Check sheet for the modelled part. Datum: model origin and axes. Units: mm. A direction names the side the tool comes from. Give positions to 0.01 mm unless a question says otherwise; leave off trailing zeros. Order: outer loops, then holes, each group sorted by start corner. A loop starts at its lowest first (then second) coordinate and runs counter-clockwise, first axis right, second up. Notation, with made-up numbers: (69, -26.75) -> (95, -26.75) arc R18 cw to (95, -7.75) -> close; hole circle Ø6 at (1, 11.5). An arc over 180 degrees is marked (long way). One line per question, with ' | ' between items.
```python
from build123d import *

# Parameters (mm, degrees)
SKETCH1_W           = 60
SKETCH1_H           = 40
SKETCH1_W_2         = 12
SKETCH1_H_2         = 2.7
BOSS_EXTRUDE1_DEPTH = 2.7


with BuildPart() as part:
    # Sketch1 → Boss-Extrude1 (new body)
    with BuildSketch(Plane(origin=(0, 0, 0), x_dir=(1, 0, 0), z_dir=(0, 1, 0))):
        Rectangle(SKETCH1_W, SKETCH1_H)
        with Locations((-12, 13.65)):
            Rectangle(SKETCH1_W_2, SKETCH1_H_2, mode=Mode.SUBTRACT)
        with Locations((12, 13.65)):
            Rectangle(SKETCH1_W_2, SKETCH1_H_2, mode=Mode.SUBTRACT)
        with Locations((12, -13.65)):
            Rectangle(SKETCH1_W_2, SKETCH1_H_2, mode=Mode.SUBTRACT)
        with Locations((-12, -13.65)):
            Rectangle(SKETCH1_W_2, SKETCH1_H_2, mode=Mode.SUBTRACT)
    extrude(amount=-BOSS_EXTRUDE1_DEPTH)


solid = part.part
```
Q1. Access from +Z, -Z, +X, -X, +Y, -Y to the whole of each face (thin tool, end or side, straight path). Record for faces 4 (the face through (0, -2.7, 0)), 5 (the face through (-12, -1, -15)).
Result sheet:
face 4: +Z, -Z, +X, -X, -Y | face 5: +Y, -Y
Q2. Thickness scan on line 1 (X direction, y = -2.2, z = 14); line 2 (Z direction, x = 14, y = -0.7). Record the ranges inside material, lowest first.
Result sheet:
line 1: x = -30 to -18, -6 to 6, 18 to 30 | line 2: z = -20 to -15, -12.3 to 12.3, 15 to 20
Q3. Section check B-B (y = -1.8). Enter the section's corners in (x, z), and give its area (3 significant figures).
Result sheet:
outline: (-30, -20) -> (30, -20) -> (30, 20) -> (-30, 20) -> close; hole (-18, -15) -> (-6, -15) -> (-6, -12.3) -> (-18, -12.3) -> close; hole (-18, 12.3) -> (-6, 12.3) -> (-6, 15) -> (-18, 15) -> close; hole (6, -15) -> (18, -15) -> (18, -12.3) -> (6, -12.3) -> close; hole (6, 12.3) -> (18, 12.3) -> (18, 15) -> (6, 15) -> close | area: 2,270 mm2
Q4. Mould release check, pull along Z, two halves, no side actions. Record for faces 1 (the face through (-12, -1, 15)), 2 (the face through (-30, -1, 0)), 3 (the face through (0, -1, -20)): pulls with the +Z half, pulls with the -Z half, needs draft (parallel to the pull), parting line crosses it, or undercut.
Result sheet:
face 1: undercut | face 2: needs draft | face 3: pulls with the -Z half
Q5. Section check A-A (x = -16). Enter the section's corners in (y, z), and give its area (3 significant figures).
Result sheet:
outline: (-2.7, -20) -> (0, -20) -> (0, -15) -> (-2.7, -15) -> close; (-2.7, -12.3) -> (0, -12.3) -> (0, 12.3) -> (-2.7, 12.3) -> close; (-2.7, 15) -> (0, 15) -> (0, 20) -> (-2.7, 20) -> close | area: 93.4 mm2
